```python
from build123d import *

# Parameters (mm, degrees)
F1_DEPTH = 25


with BuildPart() as f1:
    # F0 (on Front) → F1 (new body)
    with BuildSketch(Plane.XZ):
        with BuildLine():
            Line((44.989612, 51.928312), (-56.628712, 51.928312))
            Line((-56.628712, 51.928312), (-56.628712, 30.440735))
            Line((-56.628712, 30.440735), (-79.459257, 30.440735))
            Line((-79.459257, 30.440735), (-79.459257, -29.99307))
            Line((-79.459257, -29.99307), (-57.971686, -29.99307))
            Line((-57.971686, -29.99307), (-57.971686, -52.375961))
            Line((-57.971686, -52.375961), (44.094294, -52.375961))
            Line((44.094294, -52.375961), (44.094294, -29.99307))
            ThreePointArc((44.094294, -29.99307), (1.06181, 3.941063), (44.989612, 36.707941))
            Line((44.989612, 36.707941), (44.989612, 51.928312))
        make_face()
    extrude(amount=F1_DEPTH)


solid = f1.part
```
Geometry check sheet. Reference: the model listing, model coordinates, mm. A direction names the side the tool comes from. Round coordinates to 2 decimals unless told otherwise and drop trailing zeros. Loops run counter-clockwise (first coordinate to the right, second up) from the corner with the lowest first, then second, coordinate; pieces in that order, holes last. Notation, with made-up numbers: (-9, 25.25) - (46, 25.25) arc R24 cw to (46, 44.25) - close; hole circle Ø9 at (78, 27). An arc over 180 degrees is marked (long way). Write item = value, one per line. Start each with the question number.
1. Set-up check for faces 5 (the face through (-18, 0, 1)), 6 (the face through (44.094, -12, -41)), 7 (the face through (-69, -12, -29.993)), 8 (the face through (-68, -12, 30.441)): record each of +Z, -Z, +X, -X, +Y, -Y from which the full face is reachable in a straight line by a thin tool's end or side.
2. Mould release check, pull along X, two halves, no side actions. Record for faces 1 (the face through (44.99, -12, 44)), 2 (the face through (-57.972, -12, -41)), 3 (the face through (1.06, -12.32, 3.05)), 4 (the face through (-5, -12, 51.928)): released by +X, released by -X, zero draft, split by the parting line, or undercut.
3. Section check B-B on y = -3. Enter the section's corners in (x, z), then the cut area to 3 significant figures.
4. Section check D-D on z = -25.5. Enter the section's corners in (x, y).
5. Thickness scan on line 1 (X direction, y = -3.25, z = -38.5); line 2 (Z direction, x = 21, y = -21); line 3 (Z direction, x = -74, y = -21.75). Record the ranges inside material, lowest first.
6. Section check C-C on z = -13. Enter the section's corners in (x, y), then the cut area to 3 significant figures.
7. Depth check by flat-ended pin: pin 1 (6 mm diameter, centred on x = -65.5, y = -7.5, fed in from +Z); pin 2 (6.5 mm diameter, centred on y = -13.5, z = 36, fed in from -X). Enter the tip coordinate at first touch or a pass-through.
8. Section check A-A on x = 14.5. Enter the section's corners in (y, z), then the cut area to 3 significant figures.
Working result:
q1.face_5 = +Z, -Z, +X, -X, +Y
q1.face_6 = -Z, +X, +Y, -Y
q1.face_7 = -Z, -X, +Y, -Y
q1.face_8 = +Z, -X, +Y, -Y
q2.face_1 = released by +X
q2.face_2 = released by -X
q2.face_3 = undercut
q2.face_4 = zero draft
q3.outline = (-79.46, -29.99) - (-57.97, -29.99) - (-57.97, -52.38) - (44.09, -52.38) - (44.09, -29.99) arc R34.53 cw (long way) to (44.99, 36.71) - (44.99, 51.93) - (-56.63, 51.93) - (-56.63, 30.44) - (-79.46, 30.44) - close
q3.area = 9,470 mm^2
q4.outline = (-79.46, -25) - (16.81, -25) - (16.81, 0) - (-79.46, 0) - close
q5.line_1 = -57.97 to 44.09
q5.line_2 = -52.38 to -27.82, 34.78 to 51.93
q5.line_3 = -29.99 to 30.44
q6.outline = (-79.46, -25) - (5.24, -25) - (5.24, 0) - (-79.46, 0) - close
q6.area = 2,120 mm^2
q7.pin_1 = 30.44
q7.pin_2 = -56.63
q8.outline = (-25, -52.38) - (0, -52.38) - (0, -23.87) - (-25, -23.87) - close; (-25, 30.82) - (0, 30.82) - (0, 51.93) - (-25, 51.93) - close
q8.area = 1,240 mm^2
